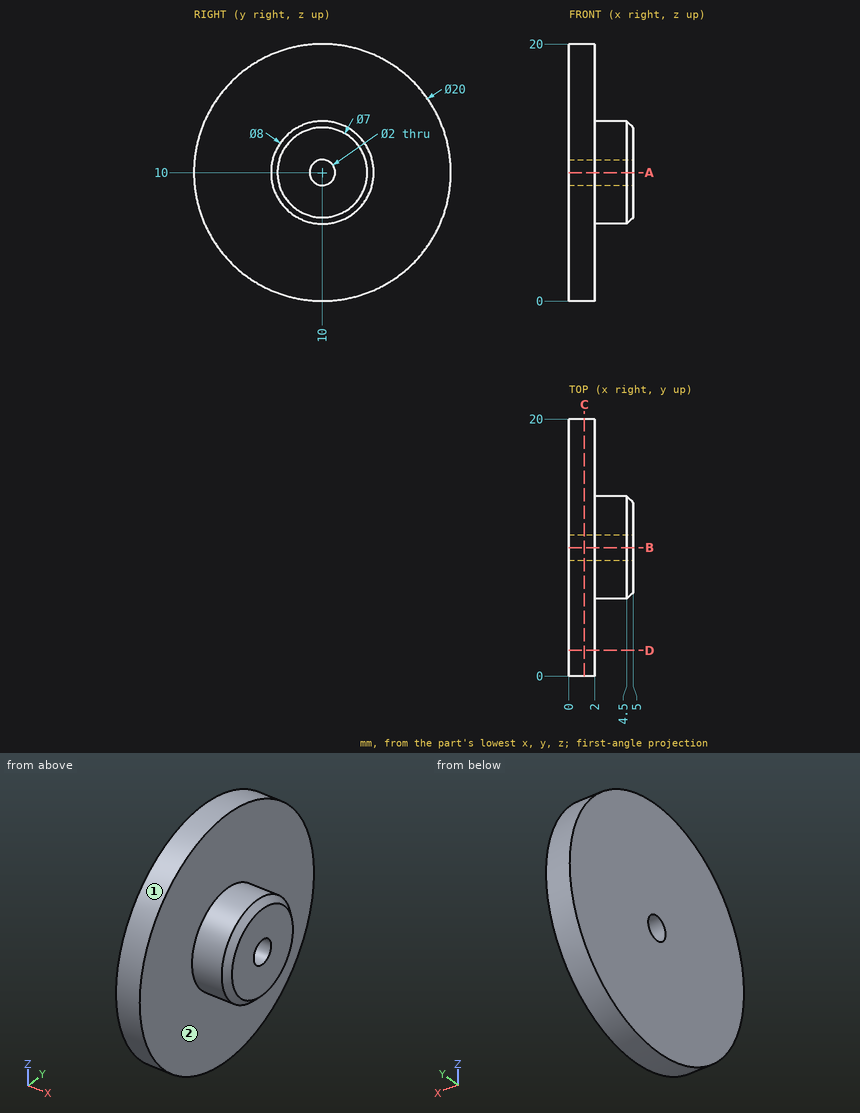
Geometry: see drawing. Coordinates: mm, zero at the bounding-box minimum. A direction names the side the tool comes from. Round coordinates to 2 decimals unless told otherwise and drop trailing zeros. Loops run counter-clockwise (first coordinate to the right, second up) from the corner with the lowest first, then second, coordinate; pieces in that order, holes last. Notation, with made-up numbers: (76.5, 59.25) -> (125.5, 59.25) arc R16 ccw to (125.5, 68.25) -> close; hole circle Ø11 at (-2, 71). An arc over 180 degrees is marked (long way). One line per question, with ' | ' between items. Start each with the question number.
1. Line query: line 1 along Z through (x, y) = (2.15, 10); line 2 along X through (y, z) = (15.25, 10.5); line 3 along Y through (x, z) = (0.45, 10.75). Output: solid intervals per line, ascending. Write a range as [from, to].
2. Section A-A on z = 10. Output: boundary loops of the cut face in (x, y).
3. Section C-C on x = 1.2. Output: boundary loops of the cut face in (y, z).
4. Section D-D on y = 2. Output: boundary loops of the cut face in (x, z).
5. Set-up query: the marked faces 1 and 2. Return all of +Z, -Z, +X, -X, +Y, -Y with unobstructed straight access to the full face (end or side cutting, diameter ignored); none if empty.
6. Contact query for flat-ended pins moving along their axis: pin 1 (2 mm diameter, centred on x = 1.5, z = 4, fed in from +Y); pin 2 (1 mm diameter, centred on y = 3.5, z = 11, fed in from +X); pin 3 (2 mm diameter, centred on x = 2.5, y = 13.5, fed in from -Z). Output: stop coordinate, or through.
Returned:
1) line 1: z = [6, 9], [11, 14] | line 2: x = [0, 2] | line 3: y = [0.03, 9.34], [10.66, 19.97]
2) outline: (0, 0) -> (2, 0) -> (2, 6) -> (4.5, 6) -> (5, 6.5) -> (5, 9) -> (0, 9) -> close; (0, 11) -> (5, 11) -> (5, 13.5) -> (4.5, 14) -> (2, 14) -> (2, 20) -> (0, 20) -> close
3) outline: circle Ø20 at (10, 10); hole circle Ø2 at (10, 10)
4) outline: (0, 4) -> (2, 4) -> (2, 16) -> (0, 16) -> close
5) face 1: +X, -X | face 2: +X
6) pin 1: stops at y = 18.66 | pin 2: stops at x = 2 | pin 3: stops at z = 0.35
